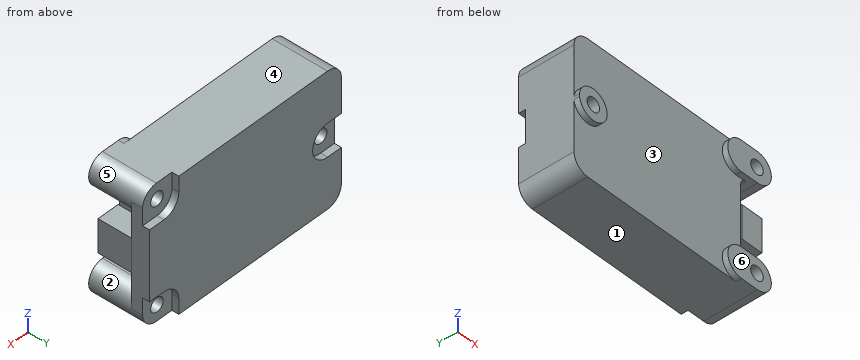
from build123d import *

# Parameters (mm, degrees)
SKIZZE1_R                       = 1.25
AUFSATZ_LINEAR_AUSTRAGEN1_DEPTH = 11
SCHNITT_LINEAR_AUSTRAGEN1_DEPTH = 1.25
SKIZZE3_OUTSIDE_W               = 49.38
SKIZZE3_OUTSIDE_H               = 35.38
SKIZZE3_OUTSIDE_R               = 2.75
SCHNITT_LINEAR_AUSTRAGEN2_DEPTH = 1
SCHNITT_LINEAR_AUSTRAGEN3_DEPTH = 6.7
SKIZZE5_W                       = 4
SKIZZE5_H                       = 6
AUFSATZ_LINEAR_AUSTRAGEN2_DEPTH = 6


with BuildPart() as part:
    # Skizze1 → Aufsatz-Linear austragen1 (new body)
    with BuildSketch(Plane(origin=(0, 0, 0), x_dir=(1, 0, 0), z_dir=(0, 1, 0))):
        with BuildLine():
            Line((-19.05, -9.31), (-19.05, 9.31))
            ThreePointArc((-19.05, 9.31), (-18.24747258, 11.24747258), (-16.31, 12.05))
            Line((-16.31, 12.05), (16.31, 12.05))
            ThreePointArc((16.31, 12.05), (18.24747258, 11.24747258), (19.05, 9.31))
            Line((19.05, 9.31), (19.05, -9.31))
            ThreePointArc((19.05, -9.31), (18.24747258, -11.24747258), (16.31, -12.05))
            Line((16.31, -12.05), (-16.31, -12.05))
            ThreePointArc((-16.31, -12.05), (-18.24747258, -11.24747258), (-19.05, -9.31))
        make_face()
        with Locations((16.2, 9.245)):
            Circle(SKIZZE1_R, mode=Mode.SUBTRACT)
        with Locations((16.2, -9.245)):
            Circle(SKIZZE1_R, mode=Mode.SUBTRACT)
        with Locations((-16.31, 0)):
            Circle(SKIZZE1_R, mode=Mode.SUBTRACT)
    extrude(amount=AUFSATZ_LINEAR_AUSTRAGEN1_DEPTH)

    # Skizze2 → Schnitt-Linear austragen1 (cut)
    with BuildSketch(Plane(origin=(0, 11, 0), x_dir=(1, 0, 0), z_dir=(0, 1, 0))):
        with BuildLine():
            Line((-19.05, -2.96), (-19.05, 2.96))
            Line((-19.05, 2.96), (-16.31, 2.96))
            ThreePointArc((-16.31, 2.96), (-13.35, 0), (-16.31, -2.96))
            Line((-16.31, -2.96), (-19.05, -2.96))
        make_face()
        with BuildLine():
            Line((13.24, 12.05), (13.24, 9.245))
            ThreePointArc((13.24, 9.245), (14.106963928, 7.151963928), (16.2, 6.285))
            Line((16.2, 6.285), (19.05, 6.285))
            Line((19.05, 6.285), (19.05, 12.05))
            Line((19.05, 12.05), (13.24, 12.05))
        make_face()
        with BuildLine():
            Line((19.05, -12.05), (13.24, -12.05))
            Line((13.24, -12.05), (13.24, -9.245))
            ThreePointArc((13.24, -9.245), (14.106963928, -7.151963928), (16.2, -6.285))
            Line((16.2, -6.285), (19.05, -6.285))
            Line((19.05, -6.285), (19.05, -12.05))
        make_face()
    extrude(amount=-SCHNITT_LINEAR_AUSTRAGEN1_DEPTH, mode=Mode.SUBTRACT)

    # Skizze3 outside → Schnitt-Linear austragen2 (cut)
    with BuildSketch(Plane.XZ):
        Rectangle(SKIZZE3_OUTSIDE_W, SKIZZE3_OUTSIDE_H)
        with Locations((-16.31, 0)):
            Circle(SKIZZE3_OUTSIDE_R, mode=Mode.SUBTRACT)
        with BuildLine():
            Line((13.14, 12.05), (16.31, 12.05))
            ThreePointArc((16.31, 12.05), (19.05, 9.31), (16.31, 6.57))
            Line((16.31, 6.57), (13.14, 6.57))
            ThreePointArc((13.14, 6.57), (10.4, 9.31), (13.14, 12.05))
        make_face(mode=Mode.SUBTRACT)
        with BuildLine():
            Line((13.14, -12.05), (16.31, -12.05))
            ThreePointArc((16.31, -12.05), (19.05, -9.31), (16.31, -6.57))
            Line((16.31, -6.57), (13.14, -6.57))
            ThreePointArc((13.14, -6.57), (10.4, -9.31), (13.14, -12.05))
        make_face(mode=Mode.SUBTRACT)
    extrude(amount=-SCHNITT_LINEAR_AUSTRAGEN2_DEPTH, mode=Mode.SUBTRACT)

    # Skizze4 → Schnitt-Linear austragen3 (cut)
    with BuildSketch(Plane.XZ.offset(-1)):
        with BuildLine():
            Line((16.31, 6.57), (15.05, 6.57))
            ThreePointArc((15.05, 6.57), (14.342893219, 6.277106781), (14.05, 5.57))
            Line((14.05, 5.57), (14.05, -5.57))
            ThreePointArc((14.05, -5.57), (14.342893219, -6.277106781), (15.05, -6.57))
            Line((15.05, -6.57), (16.31, -6.57))
            ThreePointArc((16.31, -6.57), (18.24747258, -7.37252742), (19.05, -9.31))
            Line((19.05, -9.31), (19.05, 9.31))
            ThreePointArc((19.05, 9.31), (18.24747258, 7.37252742), (16.31, 6.57))
        make_face()
    extrude(amount=-SCHNITT_LINEAR_AUSTRAGEN3_DEPTH, mode=Mode.SUBTRACT)

    # Skizze5 → Aufsatz-Linear austragen2 (add)
    with BuildSketch(Plane.XZ.offset(-7.7)):
        with Locations((17.049, 0)):
            Rectangle(SKIZZE5_W, SKIZZE5_H)
    extrude(amount=AUFSATZ_LINEAR_AUSTRAGEN2_DEPTH)


solid = part.part
Read the model definition and answer for the solid it produces. Units are mm, in the model's axes. Face numbers are marked on the shaded views. A direction names the side the tool comes from. Round coordinates to 2 decimals unless told otherwise and drop trailing zeros. Write each loop counter-clockwise with the first axis right and the second up, starting at its lowest first coordinate (ties: lowest second). Pieces come first, ordered by that corner, then holes. Notation, with made-up numbers: M 79.5,-15 L 112.5,-15 A20 ccw 112.5,12 Z; hole C -31,-35.5 d8. An arc over 180 degrees is marked long. Use a Markdown table: item, result.
1) A tool of negligible diameter and unlimited length cuts with its end or side. For the marked faces 1, 2 and 3, from which of +Z, -Z, +X, -X, +Y, -Y can it reach the whole face along a straight path? Write none if from no direction.
Answers follow:
| item | result |
|---|---|
| face 1 | -Z, +X, -X, +Y, -Y |
| face 2 | +X, -Y |
| face 3 | -Y |
2) For a pull along Z with two mould halves and no side action, classify the marked faces 4, 5 and 6 as pulls with the +Z half, pulls with the -Z half, needs draft (parallel to the pull), parting line crosses it, or undercut.
Answers follow:
| item | result |
|---|---|
| face 4 | pulls with the +Z half |
| face 5 | undercut |
| face 6 | needs draft |
3) Flat-ended cylindrical pins translate along their axes: pin 1 (2 mm diameter, centred on x = -14, z = 7, fed in from -Y); pin 2 (1.4 mm diameter, centred on x = 17.5, y = 10.5, fed in from -Z) (3 decimals); pin 3 (3 mm diameter, centred on x = 15.5, z = 8.5, fed in from +Y). Find the tip coordinate at first contact, or state that the pin passes through.
Answers follow:
| item | result |
|---|---|
| pin 1 | stops at y = 1 |
| pin 2 | stops at z = -6.285 |
| pin 3 | stops at y = 9.75 |
4) The part is cut by section B-B (x = -14.5). Write down the section's boundary in (y, z), plus the area to 3 significant figures.
Answers follow:
| item | result |
|---|---|
| outline | M 0,-2.07 L 1,-2.07 L 1,-12.05 L 11,-12.05 L 11,-2.34 L 9.75,-2.34 L 9.75,2.34 L 11,2.34 L 11,12.05 L 1,12.05 L 1,2.07 L 0,2.07 Z |
| area | 239 mm2 |
5) The part is cut by section D-D (x = 0). Write down the section's boundary in (y, z), plus the area to 3 significant figures.
Answers follow:
| item | result |
|---|---|
| outline | M 1,-12.05 L 11,-12.05 L 11,12.05 L 1,12.05 Z |
| area | 241 mm2 |
6) The part is cut by section C-C (z = 4). Write down the section's boundary in (x, y), plus the area to 4 significant figures.
Answers follow:
| item | result |
|---|---|
| outline | M -19.05,1 L 14.05,1 L 14.05,7.7 L 19.05,7.7 L 19.05,11 L -19.05,11 Z |
| area | 347.5 mm2 |
7) The part is cut by section A-A (y = 6.25). Write down the section's boundary in (x, z) (3 decimals), plus the area to 3 significant figures.
Answers follow:
| item | result |
|---|---|
| outline | M -19.05,-9.31 A2.74 ccw -16.31,-12.05 L 16.31,-12.05 A2.74 ccw 16.31,-6.57 L 15.05,-6.57 A1 cw 14.05,-5.57 L 14.05,5.57 A1 cw 15.05,6.57 L 16.31,6.57 A2.74 ccw 16.31,12.05 L -16.31,12.05 A2.74 ccw -19.05,9.31 Z; M 15.049,-3 L 19.049,-3 L 19.049,3 L 15.049,3 Z; hole C -16.31,0 d2.5; hole C 16.2,-9.245 d2.5; hole C 16.2,9.245 d2.5 |
| area | 853 mm2 |
8) Straight lines are drawn through the part: line 1 along Z through (x, y) = (16.2, 7.5) (3 decimals); line 2 along X through (y, z) = (4, 0); line 3 along Z through (x, y) = (-16.31, 7.5). For each, find the intervals that lie inside material, in ascending order. Write a range as [from, to].
Answers follow:
| item | result |
|---|---|
| line 1 | z = [-12.05, -10.495], [-7.995, -6.57], [-3, 3], [6.57, 7.995], [10.495, 12.05] |
| line 2 | x = [-19.05, -17.56], [-15.06, 14.05], [15.05, 19.05] |
| line 3 | z = [-12.05, -1.25], [1.25, 12.05] |
